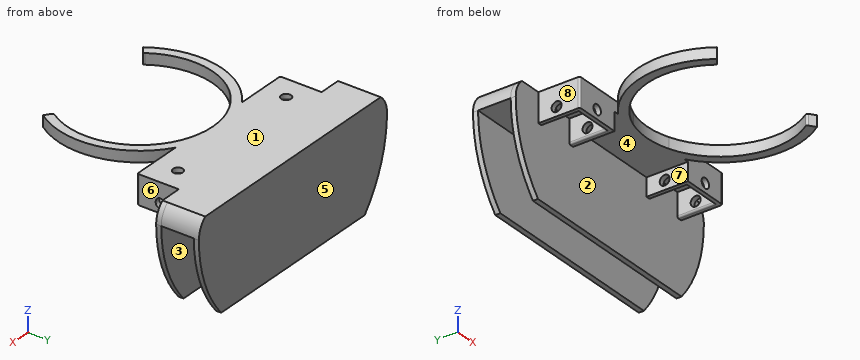
```python
from build123d import *

# Parameters (mm, degrees)
SKETCH038_W     = 105.8
SKETCH038_H     = 25.7
SKETCH038_W_2   = 20.1
SKETCH038_H_2   = 20.1
PAD020_DEPTH    = 6
SKETCH036_R     = 45.225
SKETCH036_R_2   = 40.225
PAD019_DEPTH    = 6
POCKET020_DEPTH = 6
POCKET021_DEPTH = 6
FILLET008_R     = 1
SKETCH034_W     = 25.7
SKETCH034_H     = 25.7
SKETCH034_W_2   = 20.1
SKETCH034_H_2   = 20.1
PAD021_DEPTH    = 10
SKETCH033_R     = 2.75
POCKET024_DEPTH = 105.8
SKETCH040_R     = 2.75
POCKET023_DEPTH = 2.8
FILLET009_R     = 1
PAD022_DEPTH    = 20.8
PAD018_DEPTH    = 2.8
SKETCH041_W     = 139.326154
SKETCH041_H     = 46.5
POCKET025_DEPTH = 61
SKETCH035_W     = 139.326154
SKETCH035_H     = 18
POCKET022_DEPTH = 45
SKETCH051_W     = 20.1
SKETCH051_H     = 20.1
SKETCH051_R     = 2.75
PAD028_DEPTH    = 2.8


with BuildPart() as part:
    # Sketch038 → Pad020 (new body)
    with BuildSketch(Plane.XY):
        with Locations((52.9, 12.85)):
            Rectangle(SKETCH038_W, SKETCH038_H)
        with Locations((12.85, 12.85)):
            Rectangle(SKETCH038_W_2, SKETCH038_H_2, mode=Mode.SUBTRACT)
        with Locations((92.95, 12.85)):
            Rectangle(SKETCH038_W_2, SKETCH038_H_2, mode=Mode.SUBTRACT)
    extrude(amount=PAD020_DEPTH)

    # Sketch036 → Pad019 (join)
    with BuildSketch(Plane.XY):
        with Locations((52.9, -37.955)):
            Circle(SKETCH036_R)
        with Locations((52.9, -37.955)):
            Circle(SKETCH036_R_2, mode=Mode.SUBTRACT)
    extrude(amount=PAD019_DEPTH)

    # Pad019 Face25 → Pocket020 (cut)
    with BuildSketch(Plane(origin=(52.9, 0.910232, 6), x_dir=(0, 1, 0), z_dir=(0, 0, 1))):
        with BuildLine():
            ThreePointArc((-0.910232, -13.321734), (1.359768, 0), (-0.910232, 13.321734))
            Line((-0.910232, 13.321734), (-0.910232, -13.321734))
        make_face()
    extrude(amount=-POCKET020_DEPTH, mode=Mode.SUBTRACT)

    # Sketch039 → Pocket021 (cut)
    with BuildSketch(Plane.XY):
        with BuildLine():
            Line((52.9, -37.955), (94.041911, -66.762877))
            ThreePointArc((11.758089, -66.762877), (52.9, -88.18), (94.041911, -66.762877))
            Line((52.9, -37.955), (11.758089, -66.762877))
        make_face()
    extrude(amount=POCKET021_DEPTH, mode=Mode.SUBTRACT)

    # Fillet008
    fillet008_edges = [part.edges().sort_by_distance(p)[0] for p in [
        (19.949609, -61.027112, 3),
        (85.850391, -61.027112, 3),
    ]]
    fillet(fillet008_edges, radius=FILLET008_R)

    # Sketch034 (on Face11 of Fillet008) → Pad021 (join)
    with BuildSketch(Plane(origin=(0, 0, 0), x_dir=(1, 0, 0), z_dir=(0, 0, -1))):
        with Locations((12.85, -12.85)):
            Rectangle(SKETCH034_W, SKETCH034_H)
        with Locations((12.85, -12.85)):
            Rectangle(SKETCH034_W_2, SKETCH034_H_2, mode=Mode.SUBTRACT)
        with Locations((92.95, -12.85)):
            Rectangle(SKETCH034_W, SKETCH034_H)
        with Locations((92.95, -12.85)):
            Rectangle(SKETCH034_W_2, SKETCH034_H_2, mode=Mode.SUBTRACT)
    extrude(amount=PAD021_DEPTH)

    # Sketch033 (on Face27 of Pad021) → Pocket024 (cut)
    with BuildSketch(Plane(origin=(0, 0, 0), x_dir=(0, -1, 0), z_dir=(-1, 0, 0))):
        with Locations((-12.85, -5)):
            Circle(SKETCH033_R)
    extrude(amount=-POCKET024_DEPTH, mode=Mode.SUBTRACT)

    # Sketch040 (on Face13 of Pocket024) → Pocket023 (cut)
    with BuildSketch(Plane.XZ):
        with Locations((12.85, -5)):
            Circle(SKETCH040_R)
        with Locations((92.95, -5)):
            Circle(SKETCH040_R)
    extrude(amount=-POCKET023_DEPTH, mode=Mode.SUBTRACT)

    # Fillet009
    fillet009_edges = [part.edges().sort_by_distance(p)[0] for p in [
        (103, 12.85, -10),
        (92.95, 2.8, -10),
        (82.9, 12.85, -10),
        (22.9, 12.85, -10),
        (12.85, 2.8, -10),
        (2.8, 12.85, -10),
        (0, 0, -5),
        (0, 0, 3),
        (105.8, 0, -5),
        (105.8, 0, 3),
    ]]
    fillet(fillet009_edges, radius=FILLET009_R)

    # Sketch037 (on Face12 of Fillet009) → Pad022 (join)
    with BuildSketch(Plane(origin=(0, 25.7, 0), x_dir=(-1, 0, 0), z_dir=(0, 1, 0))):
        with BuildLine():
            Line((12.1, 6), (-117.9, 6))
            ThreePointArc((-117.9, 6), (-121.340012, 1.51689), (-122.563077, -4))
            ThreePointArc((-122.563077, -4), (-52.9, -73.663077), (16.763077, -4))
            ThreePointArc((16.763077, -4), (15.540012, 1.51689), (12.1, 6))
        make_face()
    extrude(amount=PAD022_DEPTH)

    # Pad022 Face4 → Pad018 (add)
    with BuildSketch(Plane(origin=(52.9, 25.7, -32.391454), x_dir=(-1, 0, 0), z_dir=(0, -1, 0))):
        with BuildLine():
            ThreePointArc((65, -38.391454), (68.440012, -33.908343), (69.663077, -28.391454))
            ThreePointArc((69.663077, -28.391454), (0, 41.271623), (-69.663077, -28.391454))
            ThreePointArc((-69.663077, -28.391454), (-68.440012, -33.908343), (-65, -38.391454))
            Line((-65, -38.391454), (-52.9, -38.391454))
            Line((-52.9, -38.391454), (-52.9, -32.391454))
            Line((-52.9, -32.391454), (-52.9, -22.391454))
            Line((-52.9, -22.391454), (-27.2, -22.391454))
            Line((-27.2, -22.391454), (-27.2, -32.391454))
            Line((-27.2, -32.391454), (27.2, -32.391454))
            Line((27.2, -32.391454), (27.2, -22.391454))
            Line((27.2, -22.391454), (52.9, -22.391454))
            Line((52.9, -22.391454), (52.9, -32.391454))
            Line((52.9, -32.391454), (52.9, -38.391454))
            Line((52.9, -38.391454), (65, -38.391454))
        make_face()
    extrude(amount=PAD018_DEPTH)

    # Sketch041 → Pocket025 (cut)
    with BuildSketch(Plane.XY.offset(-49)):
        with Locations((52.9, 23.25)):
            Rectangle(SKETCH041_W, SKETCH041_H)
    extrude(amount=-POCKET025_DEPTH, mode=Mode.SUBTRACT)

    # Sketch035 (on Face28 of Pocket025) → Pocket022 (cut)
    with BuildSketch(Plane(origin=(0, 0, -49), x_dir=(1, 0, 0), z_dir=(0, 0, -1))):
        with Locations((52.9, -34.7)):
            Rectangle(SKETCH035_W, SKETCH035_H)
    extrude(amount=-POCKET022_DEPTH, mode=Mode.SUBTRACT)

    # Sketch051 (on Face5 of Pocket022) → Pad028 (join)
    with BuildSketch(Plane.XY.offset(6)):
        with Locations((12.85, 12.85)):
            Rectangle(SKETCH051_W, SKETCH051_H)
        with Locations((12.85, 12.85)):
            Circle(SKETCH051_R, mode=Mode.SUBTRACT)
        with Locations((92.95, 12.85)):
            Rectangle(SKETCH051_W, SKETCH051_H)
        with Locations((92.95, 12.85)):
            Circle(SKETCH051_R, mode=Mode.SUBTRACT)
    extrude(amount=-PAD028_DEPTH)


with BuildPart() as part_1:
    # Body006 placement: moved
    add(part.part.moved(Location((1000, 0, 40))))


solid = part_1.part
```
Here's how the part is built. I have some questions about the finished solid (model axes, mm). Face numbers are marked on the shaded views. A direction names the side the tool comes from. Coordinates: 2 decimals unless noted, no trailing zeros. Order: outer loops, then holes, each group sorted by start corner. A loop starts at its lowest first (then second) coordinate and runs counter-clockwise, first axis right, second up. Notation, with made-up numbers: M -17.75,43.25 L 23.25,43.25 A28 ccw 23.25,74.25 Z; hole C -25,55 d5. An arc over 180 degrees is marked long. Answer as a JSON object with one key per item and string values. Group by question number.
(1) Suppose I cut it at C-C, the plane x = 1049.5. Please give me the cut outline in (y, z).
(2) Suppose I cut it at D-D, the plane y = 12.85. State how many separate pieces and enclosed holes the cut face has, then the cut area to 3 significant figures.
(3) Suppose I cut it at A-A, the plane y = -8. Please give me the cut outline in (x, z).
(4) If we mould it in two halves opening along X, with no side actions, what happens to the marked faces 5, 6, 7 and 8? For each: released by +X, released by -X, zero draft, split by the parting line, or undercut.
(5) I need wall thicknesses on probe 1 along Y at (x, z) = (1017, 25); probe 2 along Z at (x, y) = (1092.95, 0.9); probe 3 along X at (y, z) = (-39.5, 43.5). Which ranges of each line are inside material? Lowest first, please.
(6) For pin 1 (4.5 mm diameter, centred on y = 12.85, z = 35, fed in from -X); pin 2 (4.5 mm diameter, centred on x = 1092.95, z = 35, fed in from -Y); pin 3 (9 mm diameter, centred on y = 12.85, z = 35, fed in from -X); pin 4 (10 mm diameter, centred on y = -3, z = 34.5, fed in from +X), each with a flat end and sliding along its axis, tell me the tip position at first contact or that it passes through.
(7) Which directions (+Z, -Z, +X, -X, +Y, -Y) give clear straight access to the entire face, cutting with the end or side of a thin tool? Please do the marked faces 1, 2, 3 and 4.
(8) Suppose I cut it at B-B, the plane z = 9.5. Please give me the cut outline in (x, y).
Values found:
{
 "1": {"outline": "M 2.13,40 L 22.9,40 L 22.9,-9 L 25.7,-9 L 25.7,36 L 43.7,36 L 43.7,-9 L 46.5,-9 L 46.5,46 L 2.13,46 Z"},
 "2": {"separate pieces": "7", "enclosed holes": "0", "area": "525 mm^2"},
 "3": {"outline": "M 1019.02,40 L 1026.05,40 L 1026.05,46 L 1019.02,46 Z; M 1079.75,40 L 1086.78,40 L 1086.78,46 L 1079.75,46 Z"},
 "4": {"face 5": "zero draft", "face 6": "released by +X", "face 7": "undercut", "face 8": "released by -X"},
 "5": {"probe 1": "y = 22.9 to 25.7, 43.7 to 46.5", "probe 2": "z = 30 to 32.25, 37.75 to 46", "probe 3": "x = 1007.7 to 1012.7, 1093.1 to 1098.1"},
 "6": {"pin 1": "passes through", "pin 2": "stops at y = 22.9", "pin 3": "stops at x = 1000", "pin 4": "stops at x = 1105.8"},
 "7": {"face 1": "+Z, +X, -X, +Y, -Y", "face 2": "-Z", "face 3": "-Z, +X, -X", "face 4": "-Z, -Y"},
 "8": {"outline": "M 988.47,22.9 L 1117.33,22.9 L 1117.33,25.7 L 988.47,25.7 Z; M 988.47,43.7 L 1117.33,43.7 L 1117.33,46.5 L 988.47,46.5 Z"}
}
